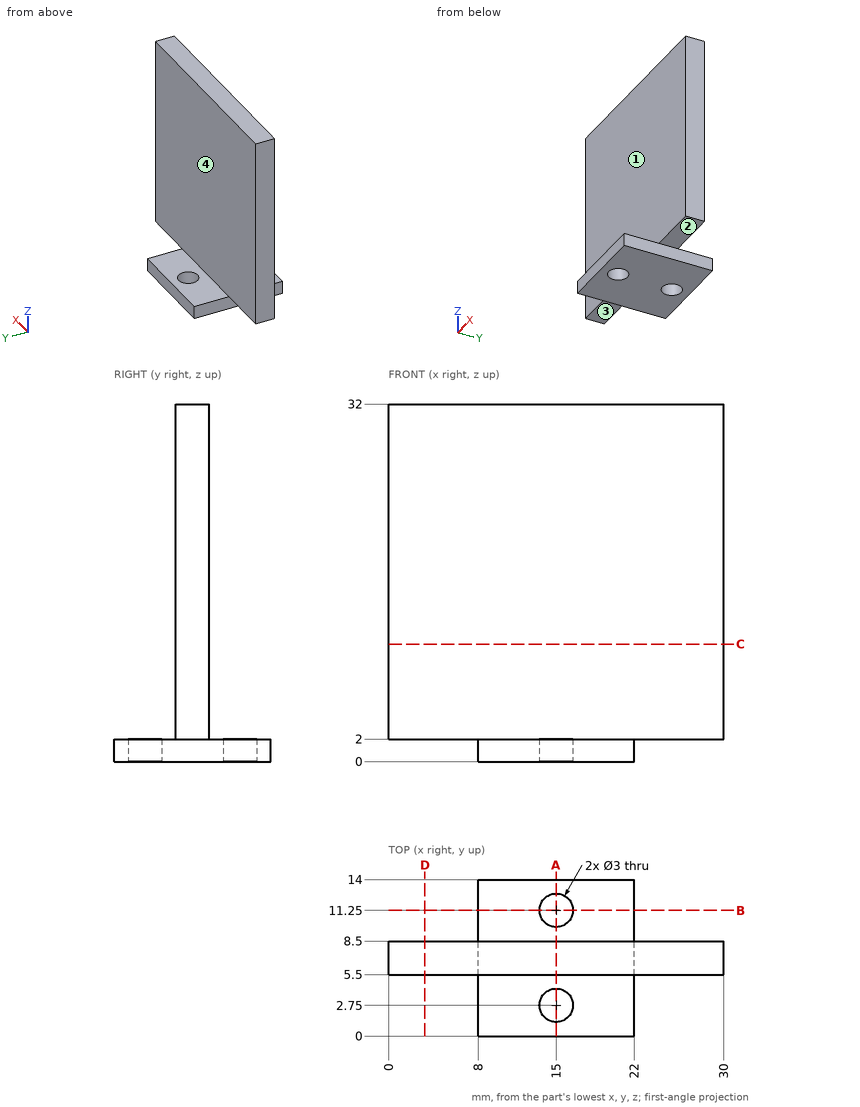
Geometry check sheet. Reference: drawing and pictorial views, mm from the part's lowest x, y, z. A direction names the side the tool comes from. Give positions to 0.01 mm unless a question says otherwise; leave off trailing zeros. Write each loop counter-clockwise with the first axis right and the second up, starting at its lowest first coordinate (ties: lowest second). Pieces come first, ordered by that corner, then holes. Notation, with made-up numbers: (80.25, -8.5) - (134.25, -8.5) arc R14 cw to (134.25, -0.5) - close; hole circle Ø4 at (58, -6). An arc over 180 degrees is marked (long way). Put each result on its own line as item: value.
Q1. Scan lines: probe 1 along Y at (x, z) = (15, 1.25); probe 2 along Y at (x, z) = (8.5, 6.5); probe 3 along Z at (x, y) = (20, 1). Record each from-to range of solid material in increasing order. Write a range as from..to.
Result:
probe 1: 0..1.25, 4.25..9.75, 12.75..14
probe 2: 5.5..8.5
probe 3: 0..2
Q2. Set-up check for the marked faces 1, 2, 3 and 4: record each of +Z, -Z, +X, -X, +Y, -Y from which the full face is reachable in a straight line by a thin tool's end or side.
Result:
face 1: +Z, +X, -X, -Y
face 2: -Z, +X, +Y, -Y
face 3: -Z, -X, +Y, -Y
face 4: +Z, +X, -X, +Y
Q3. Section check C-C on z = 10.5. Record the cut outline in (x, y), and give its area (3 significant figures).
Result:
outline: (0, 5.5) - (30, 5.5) - (30, 8.5) - (0, 8.5) - close
area: 90.0 mm2
Q4. Depth check by flat-ended pin: P1, Ø1, axis at x = 14, z = 15.5, coming from the +Y side; P2, Ø6, axis at x = 3.5, y = 4.5, coming from the +Z side; P3, Ø1, axis at x = 26.5, y = 9.5, coming from the +Z side; P4, Ø0.9, axis at x = 27.5, y = 7.5, coming from the -Z side. Enter the tip coordinate at first touch or a pass-through.
Result:
P1: y = 8.5
P2: z = 32
P3: through
P4: z = 2
Q5. Section check B-B on y = 11.25. Record the cut outline in (x, z).
Result:
outline: (8, 0) - (13.5, 0) - (13.5, 2) - (8, 2) - close; (16.5, 0) - (22, 0) - (22, 2) - (16.5, 2) - close
Q6. Section check A-A on x = 15. Record the cut outline in (y, z), and give its area (3 significant figures).
Result:
outline: (0, 0) - (1.25, 0) - (1.25, 2) - (0, 2) - close; (4.25, 0) - (9.75, 0) - (9.75, 2) - (8.5, 2) - (8.5, 32) - (5.5, 32) - (5.5, 2) - (4.25, 2) - close; (12.75, 0) - (14, 0) - (14, 2) - (12.75, 2) - close
area: 106 mm2
Q7. Section check D-D on x = 3.25. Record the cut outline in (y, z).
Result:
outline: (5.5, 2) - (8.5, 2) - (8.5, 32) - (5.5, 32) - close
